Read the model definition and answer for the solid it produces. Units are mm, in the model's axes. A direction names the side the tool comes from. Give positions to 0.01 mm unless a question says otherwise; leave off trailing zeros. Order: outer loops, then holes, each group sorted by start corner. A loop starts at its lowest first (then second) coordinate and runs counter-clockwise, first axis right, second up. Notation, with made-up numbers: (31.5, 65.25) - (74.5, 65.25) arc R27 ccw to (74.5, 89.25) - close; hole circle Ø8 at (14, 60.5). An arc over 180 degrees is marked (long way). Write item = value, one per line.
```python
from build123d import *

# Parameters (mm, degrees)
BOSS_EXTRU_1_DEPTH      = 14.5
CONG_5_R                = 7
ESQUISSE3_R             = 4
BOSS_EXTRU_2_DEPTH      = 1
CONG_2_R                = 0.5
ESQUISSE4_R             = 2
ENL_V_MAT_EXTRU_1_DEPTH = 5
ESQUISSE5_R             = 2.375
ENL_V_MAT_EXTRU_2_DEPTH = 41
ESQUISSE6_W             = 4
ESQUISSE6_H             = 7.5
ENL_V_MAT_EXTRU_3_DEPTH = 11


with BuildPart() as part:
    # Esquisse2 → Boss.-Extru.1 (new body)
    with BuildSketch(Plane(origin=(0, 0, 0), x_dir=(1, 0, 0), z_dir=(0, 1, 0))):
        Polygon((0, 0), (0, 3.5), (20, 3.5), (20, 6.5), (40, 6.5), (40, 3.5), (22, 3.5), (22, 0), align=None)
    extrude(amount=BOSS_EXTRU_1_DEPTH)

    # Congé5
    cong_5_edges = [part.edges().sort_by_distance(p)[0] for p in [
        (40, 14.5, -5),
    ]]
    fillet(cong_5_edges, radius=CONG_5_R)

    # Esquisse3 → Boss.-Extru.2 (add)
    with BuildSketch(Plane.XY.offset(-3.5)):
        with Locations((32, 7.25)):
            Circle(ESQUISSE3_R)
    extrude(amount=BOSS_EXTRU_2_DEPTH)

    # Congé2
    cong_2_edges = [part.edges().sort_by_distance(p)[0] for p in [
        (28, 7.25, -2.5),
    ]]
    fillet(cong_2_edges, radius=CONG_2_R)

    # Esquisse4 → Enlèv. mat.-Extru.1 (cut, through all)
    with BuildSketch(Plane.XY.offset(-2.5)):
        with Locations((32, 7.25)):
            Circle(ESQUISSE4_R)
    extrude(amount=-ENL_V_MAT_EXTRU_1_DEPTH, mode=Mode.SUBTRACT)

    # Symétrie1: part across plane


with BuildPart() as part_1:
    add(part.part)
    add(part.part.mirror(Plane(origin=(22, 14.5, 0), x_dir=(1, 0, 0), z_dir=(0, 0, -1))))

    # Esquisse5 → Enlèv. mat.-Extru.2 (cut, through all)
    with BuildSketch(Plane.ZY):
        with Locations((0, 7.25)):
            Circle(ESQUISSE5_R)
    extrude(amount=-ENL_V_MAT_EXTRU_2_DEPTH, mode=Mode.SUBTRACT)

    # Esquisse6 → Enlèv. mat.-Extru.3 (cut, through all)
    with BuildSketch(Plane(origin=(0, 0, -3.5), x_dir=(-1, 0, 0), z_dir=(0, 0, -1))):
        with Locations((-6.5, 7.25)):
            Rectangle(ESQUISSE6_W, ESQUISSE6_H)
    extrude(amount=-ENL_V_MAT_EXTRU_3_DEPTH, mode=Mode.SUBTRACT)


solid = part_1.part
```
1. Section C-C (y = 1) is taken. Determine the outline of the cut face in (x, z), and give its area (3 significant figures).
Recorded:
outline = (0, -3.5) - (20, -3.5) - (20, -6.5) - (40, -6.5) - (40, -3.5) - (22, -3.5) - (22, 3.5) - (40, 3.5) - (40, 6.5) - (20, 6.5) - (20, 3.5) - (0, 3.5) - close
area = 274 mm^2
2. For faces 5 (the face through (28.826, 4.816, 3.254)), 6 (the face through (34, 6, -2.5)), 7 (the face through (10, 7, -3.5)), 8 (the face through (20, 7, 5)), determine the directions among +Z, -Z, +X, -X, +Y, -Y from which every point of the face is accessible in a straight line to the end or side of a thin tool.
Recorded:
face_5 = none
face_6 = +X, +Y, -Y
face_7 = -Z, -X, +Y, -Y
face_8 = +Z, -X, +Y, -Y
3. Determine the mould class of faces 1 (the face through (38, 12.4, 5)), 2 (the face through (2.22, 4.93, -0.51)), 3 (the face through (20, 7, -5)), 4 (the face through (33.908, 7.851, -4.472)) for opening direction Y: +Y half, -Y half, draft (parallel to the pull), parting line (faces both ways), or undercut.
Recorded:
face_1 = +Y half
face_2 = undercut
face_3 = draft
face_4 = undercut
4. Flat-ended cylindrical pins translate along their axes: pin 1 (4.5 mm diameter, centred on x = 7.5, z = 0, fed in from -Y); pin 2 (0.9 mm diameter, centred on y = 7, z = -5, fed in from -X); pin 3 (4 mm diameter, centred on y = 13, z = 2.5, fed in from +X); pin 4 (5 mm diameter, centred on x = 15, y = 11, fed in from +Z). Find the tip coordinate at first contact, or state that the pin passes through.
Recorded:
pin_1 = 0
pin_2 = 20
pin_3 = 38.9
pin_4 = 3.5
5. Straight lines are drawn through the part: L1, parallel to Z at x = 37, y = 3.5; L2, parallel to Y at x = 1.7, z = 0 (3 decimals); L3, parallel to Y at x = 32, z = -5.15. For each, find the intervals that lie inside material, in ascending order. Write a range as [from, to].
Recorded:
L1 = [-6.5, -3.5], [3.5, 6.5]
L2 = [0, 4.875], [9.625, 14.5]
L3 = [0, 5.25], [9.25, 14.5]
6. Section A-A (z = 0) is taken. Determine the outline of the cut face in (x, y) (3 decimals).
Recorded:
outline = (0, 0) - (22, 0) - (22, 4.875) - (8.5, 4.875) - (8.5, 3.5) - (4.5, 3.5) - (4.5, 4.875) - (0, 4.875) - close; (0, 9.625) - (4.5, 9.625) - (4.5, 11) - (8.5, 11) - (8.5, 9.625) - (22, 9.625) - (22, 14.5) - (0, 14.5) - close
7. Section B-B (x = 32) is taken. Determine the outline of the cut face in (y, z).
Recorded:
outline = (0, -6.5) - (5.25, -6.5) - (5.25, -2.5) - (3.75, -2.5) arc R0.5 ccw to (3.25, -3) - (3.25, -3.5) - (0, -3.5) - close; (0, 3.5) - (3.25, 3.5) - (3.25, 3) arc R0.5 ccw to (3.75, 2.5) - (5.25, 2.5) - (5.25, 6.5) - (0, 6.5) - close; (9.25, -6.5) - (14.5, -6.5) - (14.5, -3.5) - (11.25, -3.5) - (11.25, -3) arc R0.5 ccw to (10.75, -2.5) - (9.25, -2.5) - close; (9.25, 2.5) - (10.75, 2.5) arc R0.5 ccw to (11.25, 3) - (11.25, 3.5) - (14.5, 3.5) - (14.5, 6.5) - (9.25, 6.5) - close
8. Section D-D (x = 3) is taken. Determine the outline of the cut face in (y, z) (3 decimals).
Recorded:
outline = (0, -3.5) - (14.5, -3.5) - (14.5, 3.5) - (0, 3.5) - close; hole circle Ø4.75 at (7.25, 0)
